from build123d import *

# Parameters (mm, degrees)
F0_W     = 15.25
F0_H     = 20
F0_W_2   = 11
F0_H_2   = 15.6
F1_DEPTH = 25
F2_W     = 13.1
F2_H     = 17.7
F2_W_2   = 11
F2_H_2   = 15.6
F3_DEPTH = 2.25
F4_W     = 13.1
F4_H     = 17.7
F4_W_2   = 11
F4_H_2   = 15.6
F5_DEPTH = 2.25


with BuildPart() as f1:
    # F0 (on Front) → F1 (new body)
    with BuildSketch(Plane.XZ):
        Rectangle(F0_W, F0_H)
        Rectangle(F0_W_2, F0_H_2, mode=Mode.SUBTRACT)
    extrude(amount=F1_DEPTH)

    # F2 (on face) → F3 (join)
    with BuildSketch(Plane(origin=(0, 0, 0), x_dir=(-1, 0, 0), z_dir=(0, 1, 0))):
        Rectangle(F2_W, F2_H)
        Rectangle(F2_W_2, F2_H_2, mode=Mode.SUBTRACT)
    extrude(amount=F3_DEPTH)

    # F4 (on face) → F5 (cut)
    with BuildSketch(Plane.XZ.offset(25)):
        Rectangle(F4_W, F4_H)
        Rectangle(F4_W_2, F4_H_2, mode=Mode.SUBTRACT)
    extrude(amount=-F5_DEPTH, mode=Mode.SUBTRACT)


solid = f1.part
Read the model definition and answer for the solid it produces. Units are mm, in the model's axes. A direction names the side the tool comes from. Give positions to 0.01 mm unless a question says otherwise; leave off trailing zeros. Write each loop counter-clockwise with the first axis right and the second up, starting at its lowest first coordinate (ties: lowest second). Pieces come first, ordered by that corner, then holes. Notation, with made-up numbers: (29.25, -23) - (39.25, -23) arc R18 ccw to (39.25, -14) - close; hole circle Ø2 at (84, -27). An arc over 180 degrees is marked (long way). Return JSON: item names as keys, results as strings.
Q1. A cutting plane is placed at A-A, the plane z = -2.25. Determine the outline of the cut face in (x, y) (3 decimals).
Reply:
{"outline": "(-7.625, -25) - (-6.55, -25) - (-6.55, -22.75) - (-5.5, -22.75) - (-5.5, 2.25) - (-6.55, 2.25) - (-6.55, 0) - (-7.625, 0) - close; (5.5, -22.75) - (6.55, -22.75) - (6.55, -25) - (7.625, -25) - (7.625, 0) - (6.55, 0) - (6.55, 2.25) - (5.5, 2.25) - close"}
Q2. For faces 1 (the face through (0, 1, 8.85)), 2 (the face through (0, -10, -7.8)), 3 (the face through (-6, -22.75, 0)), 4 (the face through (0, 1, -8.85)), determine the directions among +Z, -Z, +X, -X, +Y, -Y from which every point of the face is accessible in a straight line to the end or side of a thin tool.
Reply:
{"face 1": "+Z, +X, -X, +Y", "face 2": "+Y, -Y", "face 3": "-Y", "face 4": "-Z, +X, -X, +Y"}
Q3. A cutting plane is placed at C-C, the plane y = -1. Determine the outline of the cut face in (x, z) (3 decimals), and give its area (3 significant figures).
Reply:
{"outline": "(-7.625, -10) - (7.625, -10) - (7.625, 10) - (-7.625, 10) - close; hole (-5.5, -7.8) - (5.5, -7.8) - (5.5, 7.8) - (-5.5, 7.8) - close", "area": "133 mm²"}
Q4. Given P1, Ø1.1, axis at y = 1.5, z = -1, coming from the +X side; P2, Ø0.7, axis at y = 1, z = 1, coming from the -X side; P3, Ø1.1, axis at x = -1.5, y = 1, coming from the +Z side, each flat-ended and moving along its own axis, determine where each tip first touches the part or whether it passes through.
Reply:
{"P1": "x = 6.55", "P2": "x = -6.55", "P3": "z = 8.85"}
Q5. A cutting plane is placed at B-B, the plane x = 5. Determine the outline of the cut face in (y, z).
Reply:
{"outline": "(-25, -10) - (0, -10) - (0, -8.85) - (2.25, -8.85) - (2.25, -7.8) - (-22.75, -7.8) - (-22.75, -8.85) - (-25, -8.85) - close; (-25, 8.85) - (-22.75, 8.85) - (-22.75, 7.8) - (2.25, 7.8) - (2.25, 8.85) - (0, 8.85) - (0, 10) - (-25, 10) - close"}
Q6. For a pull along X with two mould halves and no side action, classify faces 5 (the face through (0, -24, 8.85)), 6 (the face through (-6.55, 1, 0)), 7 (the face through (0, -12, -10)), 8 (the face through (-6.55, -24, 0)) as released by +X, released by -X, zero draft, split by the parting line, or undercut.
Reply:
{"face 5": "undercut", "face 6": "released by -X", "face 7": "zero draft", "face 8": "undercut"}
Q7. Consider line 1 along X through (y, z) = (-17.5, -4.75) (3 decimals); line 2 along Z through (x, y) = (3, -7.25); line 3 along Y through (x, z) = (4.5, 9.25). Determine where each line is inside the solid, lowest interval first. Write a range as [from, to].
Reply:
{"line 1": "[-7.625, -5.5], [5.5, 7.625]", "line 2": "[-10, -7.8], [7.8, 10]", "line 3": "[-25, 0]"}
Q8. A cutting plane is placed at D-D, the plane z = -8.25. Determine the outline of the cut face in (x, y) (3 decimals).
Reply:
{"outline": "(-7.625, -25) - (-6.55, -25) - (-6.55, -22.75) - (6.55, -22.75) - (6.55, -25) - (7.625, -25) - (7.625, 0) - (6.55, 0) - (6.55, 2.25) - (-6.55, 2.25) - (-6.55, 0) - (-7.625, 0) - close"}
